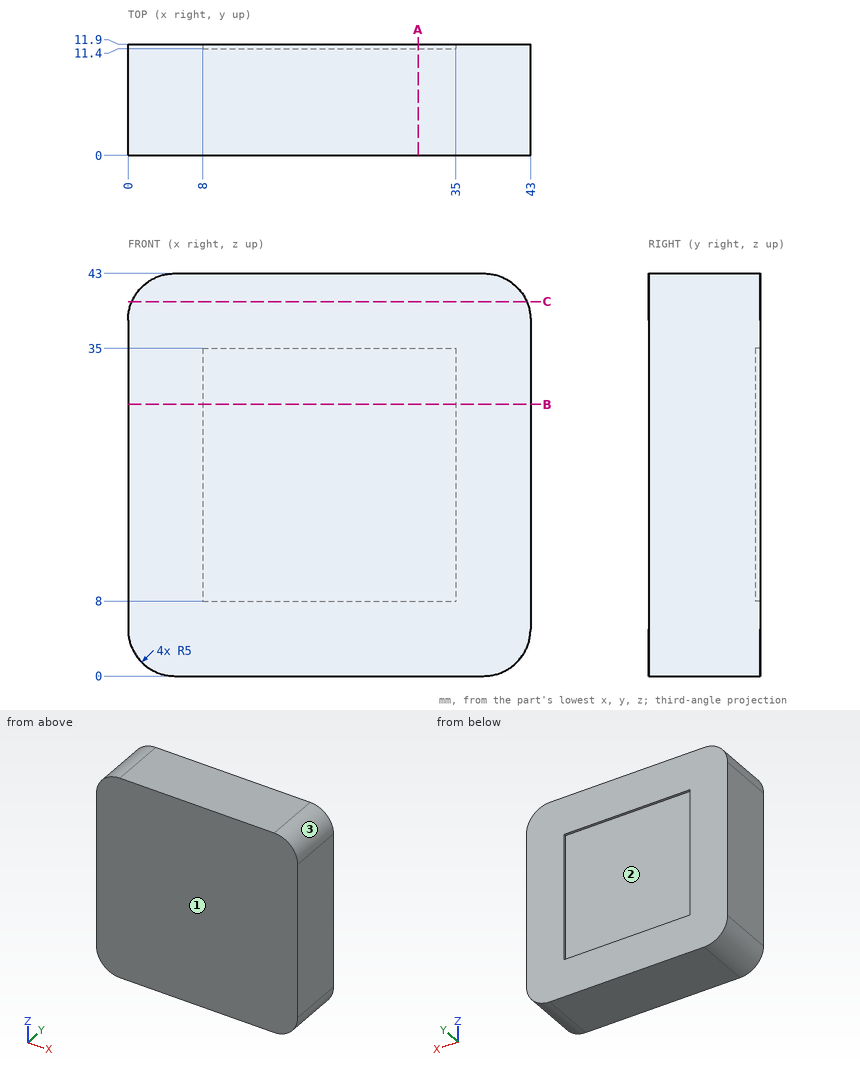
For this review, use the dimensioned drawing (mm, ordinates from the lowest corner) and the shaded views. Give positions to 0.01 mm unless a question says otherwise; leave off trailing zeros. Loops run counter-clockwise (first coordinate to the right, second up) from the corner with the lowest first, then second, coordinate; pieces in that order, holes last.
Item 1: For line 1 along Y through (x, z) = (29, 10.5); line 2 along Z through (x, y) = (4, 4.25); line 3 along Z through (x, y) = (4.5, 10.25), list the stretches that pass through material, from the lowest coordinate up.
Item 2: Draft analysis for pull direction Y (two halves, no side actions). For the marked faces 1, 2 and 3, state which applies: +Y half, -Y half, draft (parallel to the pull), parting line (faces both ways), or undercut.
Item 3: Insertion check: pin 1 (6 mm diameter, centred on x = 5, y = 7, fed in from -Z); pin 2 (13.5 mm diameter, centred on x = 20.5, z = 23, fed in from +Y). Each pin has a flat end and moves straight along its axis. Give the tip position at first contact, or say it passes through.
Item 4: Take a section at C-C, the plane z = 40. State the section outline as (x, y) points.
Item 5: Take a section at A-A, the plane x = 31. State the section outline as (y, z) points.
Item 6: Take a section at B-B, the plane z = 29. State the section outline as (x, y) points.
Calculated:
1. line 1: y = 0 to 11.4
1. line 2: z = 0.1 to 42.9
1. line 3: z = 0.03 to 42.97
2. face 1: -Y half
2. face 2: +Y half
2. face 3: draft
3. pin 1: stops at z = 0
3. pin 2: stops at y = 11.4
4. outline: (0.42, 0) - (42.58, 0) - (42.58, 11.9) - (0.42, 11.9) - close
5. outline: (0, 0) - (11.9, 0) - (11.9, 8) - (11.4, 8) - (11.4, 35) - (11.9, 35) - (11.9, 43) - (0, 43) - close
6. outline: (0, 0) - (43, 0) - (43, 11.9) - (35, 11.9) - (35, 11.4) - (8, 11.4) - (8, 11.9) - (0, 11.9) - close
